```python
from build123d import *

# Parameters (mm, degrees)
BOSS_EXTRUDE1_DEPTH = 2
BOSS_EXTRUDE2_DEPTH = 10
BOSS_EXTRUDE3_START = -107
BOSS_EXTRUDE3_DEPTH = 10


with BuildPart() as part:
    # Sketch1 → Boss-Extrude1 (new body)
    with BuildSketch(Plane.XY):
        Polygon((-33.541898883, 109.937648966), (-33.541898883, 2.937648966), (-153.541898883, 2.937648966), (-153.541898883, 12.937648966), (-53.541898883, 12.937648966), (-53.541898883, 99.937648966), (-153.541898883, 99.937648966), (-153.541898883, 109.937648966), align=None)
    extrude(amount=BOSS_EXTRUDE1_DEPTH)

    # Sketch2 → Boss-Extrude2 (add)
    with BuildSketch(Plane(origin=(0, 109.937648966, 0), x_dir=(1, 0, 0), z_dir=(0, 1, 0))):
        Polygon((-153.541898883, -2), (-33.541898883, -2), (-33.541898883, -42), align=None)
    extrude(amount=-BOSS_EXTRUDE2_DEPTH)

    # Sketch2<2> → Boss-Extrude3 (add)
    with BuildSketch(Plane(origin=(0, 109.937648966, 0), x_dir=(1, 0, 0), z_dir=(0, 1, 0)).offset(BOSS_EXTRUDE3_START)):
        Polygon((-153.541898883, -2), (-33.541898883, -2), (-33.541898883, -42), align=None)
    extrude(amount=BOSS_EXTRUDE3_DEPTH)


solid = part.part
```
Build history of the part. All positions in model axes, mm. A direction names the side the tool comes from. Give positions to 0.01 mm unless a question says otherwise; leave off trailing zeros. Loops run counter-clockwise (first coordinate to the right, second up) from the corner with the lowest first, then second, coordinate; pieces in that order, holes last.
1) Probe line 1 along Y through (x, z) = (-65.5, 4); line 2 along Z through (x, y) = (-47.5, 40.5); line 3 along Z through (x, y) = (-102, 100). List the from-to ranges inside material, lowest first.
Values follow:
line 1: y = 2.94 to 12.94, 99.94 to 109.94
line 2: z = 0 to 2
line 3: z = 0 to 19.18
2) Band-saw the part on C-C on x = -52. List the corners of the cut face in (y, z).
Values follow:
outline: (2.94, 0) - (109.94, 0) - (109.94, 35.85) - (99.94, 35.85) - (99.94, 2) - (12.94, 2) - (12.94, 35.85) - (2.94, 35.85) - close
3) Band-saw the part on A-A on x = -125. List the corners of the cut face in (y, z).
Values follow:
outline: (2.94, 0) - (12.94, 0) - (12.94, 11.51) - (2.94, 11.51) - close; (99.94, 0) - (109.94, 0) - (109.94, 11.51) - (99.94, 11.51) - close
4) 3-axis set-ups, long thin cutter, end or side, ignore diameter. For faces 4 (the face through (-33.542, 48, 1)), 5 (the face through (-43, 57, 2)): which of +Z, -Z, +X, -X, +Y, -Y reach the whole face in a straight line?
Values follow:
face 4: +Z, -Z, +X, +Y, -Y
face 5: +Z, +X, -X
5) Band-saw the part on D-D on y = 52.5. List the corners of the cut face in (x, z).
Values follow:
outline: (-53.54, 0) - (-33.54, 0) - (-33.54, 2) - (-53.54, 2) - close
6) Two-plate mould, pull along Y, no slides. Class faces 1 (the face through (-92.7, 7.87, 22.28)), 2 (the face through (-79, 109.938, 16)), 3 (the face through (-79, 12.938, 16)): released by +Y, released by -Y, zero draft, split by the parting line, or undercut.
Values follow:
face 1: zero draft
face 2: released by +Y
face 3: undercut
7) Band-saw the part on B-B on z = 26.5. List the corners of the cut face in (x, y), then the cut area to 3 significant figures.
Values follow:
outline: (-80.04, 2.94) - (-33.54, 2.94) - (-33.54, 12.94) - (-80.04, 12.94) - close; (-80.04, 99.94) - (-33.54, 99.94) - (-33.54, 109.94) - (-80.04, 109.94) - close
area: 930 mm2
8) Drop flat-ended pins along their axis: P1, Ø0.6, axis at y = 68.5, z = 1, coming from the -X side; P2, Ø22, axis at x = -47.5, y = 71, coming from the +Z side. Give the stop position or say it passes through.
Values follow:
P1: stops at x = -53.54
P2: stops at z = 2
